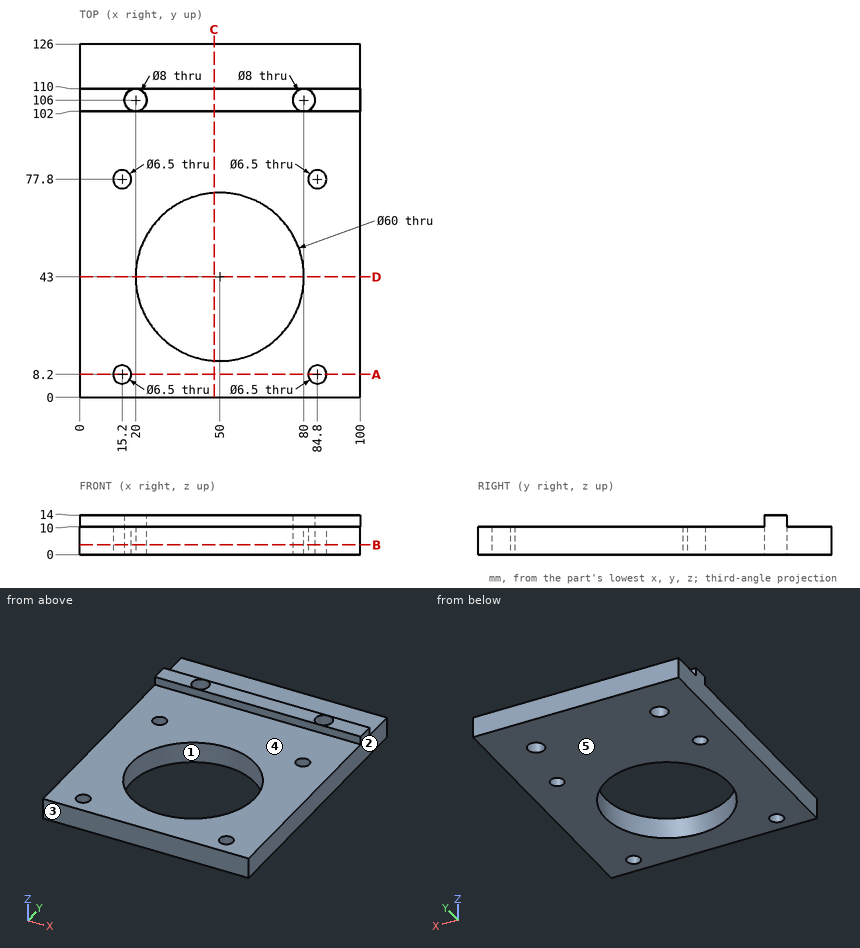
Verification items for this drawing (mm, ordinates from the low corner). A direction names the side the tool comes from. Coordinates: 2 decimals unless noted, no trailing zeros. Write each loop counter-clockwise with the first axis right and the second up, starting at its lowest first coordinate (ties: lowest second). Pieces come first, ordered by that corner, then holes. Notation, with made-up numbers: M 47.5,-12.75 L 59.5,-12.75 A16 ccw 59.5,-7.75 Z; hole C 13.25,-12 d10. An arc over 180 degrees is marked long. Use one line per item in the form item = value. Start each with the question number.
1) Section check A-A on y = 8.2. Enter the section's corners in (x, z), and give its area (3 significant figures).
2) Section check B-B on z = 3.5. Enter the section's corners in (x, y), and give its area (3 significant figures).
3) Section check C-C on x = 48. Enter the section's corners in (y, z).
4) Set-up check for the marked faces 4 and 5: record each of +Z, -Z, +X, -X, +Y, -Y from which the full face is reachable in a straight line by a thin tool's end or side.
5) Section check D-D on y = 43. Enter the section's corners in (x, z), and give its area (3 significant figures).
6) Release check for a two-part mould opening along X. For the marked faces 1, 2 and 3 record: pulls with the +X half, pulls with the -X half, needs draft (parallel to the pull), parting line crosses it, or undercut.
7) Go/stop test with flat-tipped pins: pin 1 Ø3 at (x, z) = (69.5, 12.5) entering from -Y; pin 2 Ø5 at (x, y) = (15.2, 8.2) entering from +Z; pin 3 Ø3 at (x, y) = (55, 13.5) entering from +Z. Record where each tip stops, or that it passes through.
8) Thickness scan on probe 1 along X at (y, z) = (106, 7.75); probe 2 along Y at (x, z) = (15.2, 2.75); probe 3 along Z at (x, y) = (43.5, 118). Record the ranges inside material, lowest first. Write a range as from..to.
Responses:
q1.outline = M 0,0 L 11.95,0 L 11.95,10 L 0,10 Z; M 18.45,0 L 81.55,0 L 81.55,10 L 18.45,10 Z; M 88.05,0 L 100,0 L 100,10 L 88.05,10 Z
q1.area = 870 mm2
q2.outline = M 0,0 L 100,0 L 100,126 L 0,126 Z; hole C 15.2,8.2 d6.5; hole C 15.2,77.8 d6.5; hole C 20,106 d8; hole C 50,43 d60; hole C 80,106 d8; hole C 84.8,8.2 d6.5; hole C 84.8,77.8 d6.5
q2.area = 9,540 mm2
q3.outline = M 0,0 L 13.07,0 L 13.07,10 L 0,10 Z; M 72.93,0 L 126,0 L 126,10 L 110,10 L 110,14 L 102,14 L 102,10 L 72.93,10 Z
q4.face_4 = +Z, +X, -X, -Y
q4.face_5 = -Z, +X, -X, +Y, -Y
q5.outline = M 0,0 L 20,0 L 20,10 L 0,10 Z; M 80,0 L 100,0 L 100,10 L 80,10 Z
q5.area = 400 mm2
q6.face_1 = undercut
q6.face_2 = pulls with the +X half
q6.face_3 = needs draft
q7.pin_1 = 102
q7.pin_2 = through
q7.pin_3 = 10
q8.probe_1 = 0..16, 24..76, 84..100
q8.probe_2 = 0..4.95, 11.45..74.55, 81.05..126
q8.probe_3 = 0..10
